from build123d import *

# Parameters (mm, degrees)
EXTRUDE_1_DEPTH = 10
FILLET_1_R      = 2
FILLET_2_R      = 1


with BuildPart() as part:
    # Эскиз1 → Бобышка-Вытянуть1 (new body)
    with BuildSketch(Plane.XY):
        with BuildLine():
            Line((95.45, 22.75), (95.45, 16.75))
            Line((95.45, 16.75), (104.55, 16.75))
            Line((104.55, 16.75), (104.55, 22.75))
            Line((104.55, 22.75), (106.55, 22.75))
            Line((106.55, 22.75), (106.55, 14.75))
            Line((106.55, 14.75), (4.5, -5.5))
            Line((4.5, -5.5), (-5.5, -5.5))
            Line((-5.5, -5.5), (-5.5, 0.5))
            Line((-5.5, 0.5), (-4.019017293, 0.5))
            ThreePointArc((-4.019017293, 0.5), (0, -4.05), (4.019017293, 0.5))
            Line((4.019017293, 0.5), (4.493506463, 1.63519453))
            Line((4.493506463, 1.63519453), (93.45, 19.287022008))
            Line((93.45, 19.287022008), (93.45, 22.75))
            Line((93.45, 22.75), (95.45, 22.75))
        make_face()
    extrude(amount=EXTRUDE_1_DEPTH)

    # Скругление1
    fillet_1_edges = [part.edges().sort_by_distance(p)[0] for p in [
        (4.493506463, 1.63519453, 5),
        (93.45, 19.287022008, 5),
        (106.55, 14.75, 5),
        (4.5, -5.5, 5),
        (-5.5, -5.5, 5),
    ]]
    fillet(fillet_1_edges, radius=FILLET_1_R)

    # Скругление2
    fillet_2_edges = [part.edges().sort_by_distance(p)[0] for p in [
        (93.45, 22.75, 5),
        (106.55, 22.75, 5),
        (-5.5, 0.5, 5),
    ]]
    fillet(fillet_2_edges, radius=FILLET_2_R)


solid = part.part
Source: CAD feature listing. Evaluate the final solid. Frame: model axes, mm. A direction names the side the tool comes from. Give positions to 0.01 mm unless a question says otherwise; leave off trailing zeros. Loops run counter-clockwise (first coordinate to the right, second up) from the corner with the lowest first, then second, coordinate; pieces in that order, holes last. Notation, with made-up numbers: (-28.75, -3.5) -> (-8.75, -3.5) arc R26 ccw to (-8.75, 34.5) -> close; hole circle Ø5 at (-21.75, 37). An arc over 180 degrees is marked (long way). Use a Markdown table: item, result. Add a question column.
1) Section query B-B, the plane x = 0. Return the cut outline in (y, z).
2) Section query C-C, the plane y = 10.75. Return the cut outline in (x, z).
3) Pull-direction query (X, two-part tool) for faces 3 (the face through (106.11, 15.14, 5.07)), 4 (the face through (104.55, 20, 5)), 5 (the face through (51, 7, 10)); classes: +X half, -X half, draft (parallel to the pull), parting line (faces both ways), or undercut.
4) First-contact query: pin 1 (5 mm diameter, centred on x = 0, y = 0, fed in from +Z); pin 2 (2.5 mm diameter, centred on x = 98.5, z = 4.5, fed in from +Y); pin 3 (0.9 mm diameter, centred on y = 21.5, z = 6.5, fed in from -X). Flat tips, straight axial feed; report the tip coordinate or a pass-through.
5) Line query: line 1 along Y through (x, z) = (0, 3.25); line 2 along Y through (x, z) = (59, 3). Output: solid intervals per line, ascending. Write a range as [from, to].
6) Reachability of faces 1 (the face through (106.55, 19, 5)), 2 (the face through (100, 16.75, 5)) from +Z, -Z, +X, -X, +Y, -Y: full face, straight path, thin tool, end or side. Return the list, or none.
7) Section query A-A, the plane z = 1. Return the cut outline in (x, y).
Numbers:
| question | item | result |
|---|---|---|
| 1 | outline | (-5.5, 0) -> (-4.05, 0) -> (-4.05, 10) -> (-5.5, 10) -> close |
| 2 | outline | (50.43, 0) -> (86.39, 0) -> (86.39, 10) -> (50.43, 10) -> close |
| 3 | face 3 | +X half |
| 3 | face 4 | undercut |
| 3 | face 5 | draft |
| 4 | pin 1 | passes through |
| 4 | pin 2 | stops at y = 16.75 |
| 4 | pin 3 | stops at x = 93.45 |
| 5 | line 1 | y = [-5.5, -4.05] |
| 5 | line 2 | y = [5.31, 12.45] |
| 6 | face 1 | +Z, -Z, +X, +Y, -Y |
| 6 | face 2 | +Z, -Z, +Y |
| 7 | outline | (-5.5, -3.5) arc R2 ccw to (-3.5, -5.5) -> (4.3, -5.5) arc R2 ccw to (4.69, -5.46) -> (104.94, 14.43) arc R2 ccw to (106.55, 16.39) -> (106.55, 21.75) arc R1 ccw to (105.55, 22.75) -> (104.55, 22.75) -> (104.55, 16.75) -> (95.45, 16.75) -> (95.45, 22.75) -> (94.45, 22.75) arc R1 ccw to (93.45, 21.75) -> (93.45, 20.93) arc R2 cw to (91.84, 18.97) -> (5.54, 1.84) arc R2 ccw to (4.08, 0.65) -> (4.02, 0.5) arc R4.05 cw (long way) to (-4.02, 0.5) -> (-4.5, 0.5) arc R1 ccw to (-5.5, -0.5) -> close |
